Verification items for the finished model (mm, model axes). A direction names the side the tool comes from. Round coordinates to 2 decimals unless told otherwise and drop trailing zeros. Loops run counter-clockwise (first coordinate to the right, second up) from the corner with the lowest first, then second, coordinate; pieces in that order, holes last. Notation, with made-up numbers: (-21, 72) -> (32, 72) arc R16 cw to (32, 86) -> close; hole circle Ø3 at (13.25, 73). An arc over 180 degrees is marked (long way). Write item = value, one per line.
```python
from build123d import *

# Parameters (mm, degrees)
F0_R     = 76.2
F1_DEPTH = 2000
F3_DEPTH = 670
F5_DEPTH = 61


with BuildPart() as f1:
    # F0 (on Top) → F1 (new body)
    with BuildSketch(Plane.XY):
        Circle(F0_R)
    extrude(amount=F1_DEPTH)

    # F2 (on face) → F3 (cut)
    with BuildSketch(Plane.XY.offset(2000)):
        with BuildLine():
            Line((-63.1467790732, -42.6488486677), (-76.2, -42.6488486677))
            Line((-76.2, -42.6488486677), (-76.2, -102.6488486677))
            Line((-76.2, -102.6488486677), (76.2, -102.6488486677))
            Line((76.2, -102.6488486677), (76.2, -42.6488486677))
            Line((76.2, -42.6488486677), (63.1467790732, -42.6488486677))
            ThreePointArc((63.1467790732, -42.6488486677), (0, -76.2), (-63.1467790732, -42.6488486677))
        make_face()
        with BuildLine():
            Line((63.1467790732, -42.6488486677), (-63.1467790732, -42.6488486677))
            ThreePointArc((-63.1467790732, -42.6488486677), (0, -76.2), (63.1467790732, -42.6488486677))
        make_face()
    extrude(amount=-F3_DEPTH, mode=Mode.SUBTRACT)

    # F4 (on Right) → F5 (join, symmetric)
    with BuildSketch(Plane.YZ):
        Polygon((-37.8018170595, 1330.9504985809), (-45.1709479094, 1995.6457614899), (-778.1082391739, 1684.8677396774), align=None)
    extrude(amount=F5_DEPTH, both=True)


solid = f1.part
```
(1) Material ranges on probe 1 along X at (y, z) = (-165, 1675); probe 2 along X at (y, z) = (0.5, 527.5); probe 3 along Z at (x, y) = (-54.5, -625), recorded low to high. Write a range as from..to.
Filled sheet:
probe_1 = -61..61
probe_2 = -76.2..76.2
probe_3 = 1611.67..1749.79
(2) Sectioned sample at D-D, the plane z = 790. Record the cut outline in (x, y).
Filled sheet:
outline = circle Ø152.4 at (0, 0)
(3) Sectioned sample at A-A, the plane x = 0. Record the cut outline in (y, z), and give its area (3 significant figures).
Filled sheet:
outline = (-778.11, 1684.87) -> (-42.65, 1333.27) -> (-42.65, 1330) -> (-76.2, 1330) -> (-76.2, 0) -> (76.2, 0) -> (76.2, 2000) -> (-42.65, 2000) -> (-42.65, 1768.15) -> (-45.17, 1995.65) -> close
area = 526,000 mm2
(4) Sectioned sample at C-C, the plane y = -186. Record the cut outline in (x, z), and give its area (3 significant figures).
Filled sheet:
outline = (-61, 1401.8) -> (61, 1401.8) -> (61, 1935.93) -> (-61, 1935.93) -> close
area = 65,200 mm2
(5) Sectioned sample at B-B, the plane z = 1599. Record the cut outline in (x, y), and give its area (3 significant figures).
Filled sheet:
outline = (-63.15, -42.65) -> (-61, -42.65) -> (-61, -598.49) -> (61, -598.49) -> (61, -42.65) -> (63.15, -42.65) arc R76.2 ccw (long way) to start
area = 83,100 mm2
(6) Go/stop test with flat-tipped pins: pin 1 Ø10 at (x, y) = (11, -58) entering from +Z; pin 2 Ø1 at (x, y) = (-39, -410.5) entering from +Z; pin 3 Ø4 at (x, y) = (-27, -407.5) entering from +Z. Record where each tip stops, or that it passes through.
Filled sheet:
pin_1 = 1992.33
pin_2 = 1840.95
pin_3 = 1842.86
(7) Set-up check for faces 1 (the face through (-61, -334, 1669)), 2 (the face through (61, -334, 1669)), 3 (the face through (-1, -55, 1330)), 4 (the face through (-1, 1, 0)), 5 (the face through (40.965, 64.252, 986)): record each of +Z, -Z, +X, -X, +Y, -Y from which the full face is reachable in a straight line by a thin tool's end or side.
Filled sheet:
face_1 = +Z, -Z, -X, -Y
face_2 = +Z, -Z, +X, -Y
face_3 = +X, -X, -Y
face_4 = -Z, +X, -X, +Y, -Y
face_5 = -Z
